from build123d import *

# Parameters (mm, degrees)
BOSS_EXTRUDE1_DEPTH   = 35
BOSS_EXTRUDE1_2_DEPTH = 35
BOSS_EXTRUDE2_DEPTH   = 21
SKETCH3_R             = 2
CUT_EXTRUDE1_DEPTH    = 17.585786438


with BuildPart() as part:
    # Sketch2 → Boss-Extrude1 (new body)
    with BuildSketch(Plane.XY):
        with BuildLine():
            Line((24, 18.267872099), (14, 18.267872099))
            ThreePointArc((14, 18.267872099), (12.585786438, 18.853658537), (12, 20.267872099))
            Line((12, 20.267872099), (10, 20.267872099))
            ThreePointArc((10, 20.267872099), (11.171572875, 17.439444974), (14, 16.267872099))
            Line((14, 16.267872099), (24, 16.267872099))
            Line((24, 16.267872099), (24, 18.267872099))
        make_face()
    extrude(amount=BOSS_EXTRUDE1_DEPTH)



with BuildPart() as body_2:
    # Sketch2 → Boss-Extrude1 2 (new body)
    with BuildSketch(Plane.XY):
        with BuildLine():
            Line((-24, 16.267872099), (-14, 16.267872099))
            ThreePointArc((-14, 16.267872099), (-11.171572875, 17.439444974), (-10, 20.267872099))
            Line((-10, 20.267872099), (-12, 20.267872099))
            ThreePointArc((-12, 20.267872099), (-12.585786438, 18.853658537), (-14, 18.267872099))
            Line((-14, 18.267872099), (-24, 18.267872099))
            Line((-24, 18.267872099), (-24, 16.267872099))
        make_face()
    extrude(amount=BOSS_EXTRUDE1_2_DEPTH)


with BuildPart() as part_1:
    add(part.part)

    add(body_2.part)  # Boss-Extrude2 merges body 2
    # Sketch2_3 → Boss-Extrude2 (add)
    with BuildSketch(Plane.XY):
        with BuildLine():
            Line((-24, 18.267872099), (-24, 16.267872099))
            Line((-24, 16.267872099), (-14, 16.267872099))
            ThreePointArc((-14, 16.267872099), (-11.171572875, 17.439444974), (-10, 20.267872099))
            Line((-10, 20.267872099), (-12, 20.267872099))
            ThreePointArc((-12, 20.267872099), (-12.585786438, 18.853658537), (-14, 18.267872099))
            Line((-14, 18.267872099), (-24, 18.267872099))
        make_face()
        with BuildLine():
            Line((-12, 20.267872099), (-10, 20.267872099))
            Line((-10, 20.267872099), (-10, 29.853658537))
            ThreePointArc((-10, 29.853658537), (-9.707106781, 30.560765318), (-9, 30.853658537))
            Line((-9, 30.853658537), (9, 30.853658537))
            ThreePointArc((9, 30.853658537), (9.707106781, 30.560765318), (10, 29.853658537))
            Line((10, 29.853658537), (10, 20.267872099))
            Line((10, 20.267872099), (12, 20.267872099))
            Line((12, 20.267872099), (12, 30.853658537))
            ThreePointArc((12, 30.853658537), (11.414213562, 32.267872099), (10, 32.853658537))
            Line((10, 32.853658537), (-10, 32.853658537))
            ThreePointArc((-10, 32.853658537), (-11.414213562, 32.267872099), (-12, 30.853658537))
            Line((-12, 30.853658537), (-12, 20.267872099))
        make_face()
        with BuildLine():
            Line((12, 20.267872099), (10, 20.267872099))
            ThreePointArc((10, 20.267872099), (11.171572875, 17.439444974), (14, 16.267872099))
            Line((14, 16.267872099), (24, 16.267872099))
            Line((24, 16.267872099), (24, 18.267872099))
            Line((24, 18.267872099), (14, 18.267872099))
            ThreePointArc((14, 18.267872099), (12.585786438, 18.853658537), (12, 20.267872099))
        make_face()
    extrude(amount=BOSS_EXTRUDE2_DEPTH)

    # Sketch3 → Cut-Extrude1 (cut, through all)
    with BuildSketch(Plane(origin=(0, 32.853658537, 0), x_dir=(1, 0, 0), z_dir=(0, 1, 0))):
        with Locations((0, -8)):
            Circle(SKETCH3_R)
        with Locations((0, -16)):
            Circle(SKETCH3_R)
        with Locations((-19, -5)):
            Circle(SKETCH3_R)
        with Locations((-19, -30)):
            Circle(SKETCH3_R)
        with Locations((19, -30)):
            Circle(SKETCH3_R)
        with Locations((19, -5)):
            Circle(SKETCH3_R)
    extrude(amount=-CUT_EXTRUDE1_DEPTH, mode=Mode.SUBTRACT)


solid = part_1.part
Work out the finished part from the listing and answer in its coordinate system (mm). A direction names the side the tool comes from. Coordinates: 2 decimals unless noted, no trailing zeros. Write each loop counter-clockwise with the first axis right and the second up, starting at its lowest first coordinate (ties: lowest second). Pieces come first, ordered by that corner, then holes. Notation, with made-up numbers: M 15.5,12.5 L 38.5,12.5 A23 cw 38.5,32.5 Z; hole C 81.25,-21 d8. An arc over 180 degrees is marked long. Use one line per item in the form item = value. Start each with the question number.
1. A tool of negligible diameter and unlimited length cuts with its end or side. For faces 1 (the face through (-20.6, 17.3, 6.2)), 2 (the face through (19, 18.268, 17)), 3 (the face through (-11, 20.268, 28)), 4 (the face through (-11.2, 17.41, 17.26)), 5 (the face through (-12, 26, 10)), from which of +Z, -Z, +X, -X, +Y, -Y can it reach the whole face along a straight path? Write none if from no direction.
2. The part is cut by section A-A (z = 8). Give the vertices of the cut face in (x, y).
3. The part is cut by section B-B (x = 0). Give the vertices of the cut face in (y, z), plus the area to 3 significant figures.
4. The part is cut by section D-D (y = 29). Give the vertices of the cut face in (x, z).
5. Each of these flat-tipped pins is pushed along its axis until it touches: P1, Ø8, axis at x = -18, z = 14.5, coming from the +Y side; P2, Ø3, axis at y = 25.5, z = 14, coming from the -X side; P3, Ø4, axis at y = 30.5, z = 5, coming from the +X side; P4, Ø4.5, axis at x = 19, z = 30, coming from the -Y side. Where does it stop, or does it pass through?
6. The mould has two halves that part along Z. Classify faces 6 (the face through (19, 17, 32)), 7 (the face through (12.6, 18.84, 17.26)), 8 (the face through (17, 17, 35)): released by +Z, released by -Z, zero draft, split by the parting line, or undercut.
7. The part is cut by section C-C (z = 30). Give the vertices of the cut face in (x, y), plus the area to 3 significant figures.
8. Straight lines are drawn through the part: probe 1 along Z at (x, y) = (19, 17.65); probe 2 along Z at (x, y) = (0, 31.9); probe 3 along X at (y, z) = (21, 8). For each, find the intervals that lie inside material, in ascending order. Write a range as from..to.
Evaluation:
q1.face_1 = +Y, -Y
q1.face_2 = +Z, -Z, +X, +Y
q1.face_3 = +Z, +X, -X, +Y
q1.face_4 = +Z, -Z, -Y
q1.face_5 = +Z, -Z, -X, +Y
q2.outline = M -24,16.27 L -14,16.27 A4 ccw -10,20.27 L -10,29.85 A1 cw -9,30.85 L -2,30.85 L -2,32.85 L -10,32.85 A2 ccw -12,30.85 L -12,20.27 A2 cw -14,18.27 L -24,18.27 Z; M 2,30.85 L 9,30.85 A1 cw 10,29.85 L 10,20.27 A4 ccw 14,16.27 L 24,16.27 L 24,18.27 L 14,18.27 A2 cw 12,20.27 L 12,30.85 A2 ccw 10,32.85 L 2,32.85 Z
q3.outline = M 30.85,0 L 32.85,0 L 32.85,6 L 30.85,6 Z; M 30.85,10 L 32.85,10 L 32.85,14 L 30.85,14 Z; M 30.85,18 L 32.85,18 L 32.85,21 L 30.85,21 Z
q3.area = 26.0 mm^2
q4.outline = M -12,0 L -10,0 L -10,21 L -12,21 Z; M 10,0 L 12,0 L 12,21 L 10,21 Z
q5.P1 = 18.27
q5.P2 = -12
q5.P3 = 12
q5.P4 = 16.27
q6.face_6 = undercut
q6.face_7 = zero draft
q6.face_8 = released by +Z
q7.outline = M -24,16.27 L -21,16.27 L -21,18.27 L -24,18.27 Z; M -17,16.27 L -14,16.27 A4 ccw -10,20.27 L -12,20.27 A2 cw -14,18.27 L -17,18.27 Z; M 10,20.27 A4 ccw 14,16.27 L 17,16.27 L 17,18.27 L 14,18.27 A2 cw 12,20.27 Z; M 21,16.27 L 24,16.27 L 24,18.27 L 21,18.27 Z
q7.area = 42.8 mm^2
q8.probe_1 = 0..3, 7..28, 32..35
q8.probe_2 = 0..6, 10..14, 18..21
q8.probe_3 = -12..-10, 10..12
